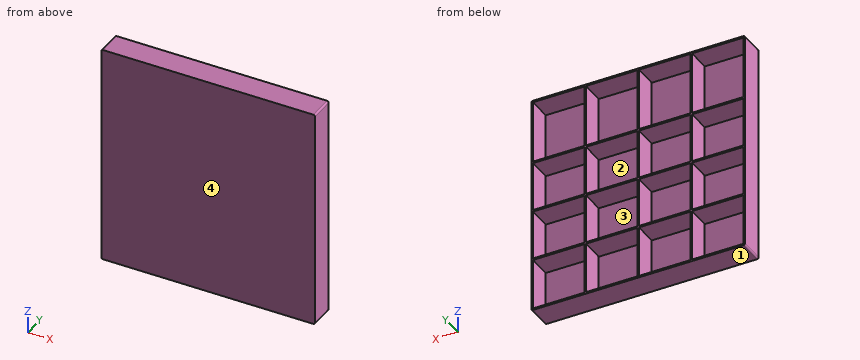
from build123d import *

# Parameters (mm, degrees)
SKETCH_1_W             = 258
SKETCH_1_H             = 268
EXTRUDE_1_DEPTH        = 2
SKETCH_2_W             = 258
SKETCH_2_H             = 268
SKETCH_2_W_2           = 254
SKETCH_2_H_2           = 264
EXTRUDE_2_DEPTH        = 28
SKETCH_3_W             = 2
SKETCH_3_H             = 264
EXTRUDE_3_DEPTH        = 28
PATTERN_LINEAR_1_COUNT = 3
PATTERN_LINEAR_1_PITCH = 64
SKETCH_4_W             = 254
SKETCH_4_H             = 2
EXTRUDE_5_DEPTH        = 28
PATTERN_LINEAR_2_COUNT = 3
PATTERN_LINEAR_2_PITCH = 62
FILLET_1_R             = 2


with BuildPart() as part:
    # 草图1 → 凸台-拉伸1 (new body)
    with BuildSketch(Plane(origin=(0, 0, 0), x_dir=(1, 0, 0), z_dir=(0, 1, 0))):
        Rectangle(SKETCH_1_W, SKETCH_1_H)
    extrude(amount=EXTRUDE_1_DEPTH)

    # 草图2 → 凸台-拉伸2 (add)
    with BuildSketch(Plane(origin=(0, 2, 0), x_dir=(1, 0, 0), z_dir=(0, 1, 0))):
        Rectangle(SKETCH_2_W, SKETCH_2_H)
        Rectangle(SKETCH_2_W_2, SKETCH_2_H_2, mode=Mode.SUBTRACT)
    extrude(amount=EXTRUDE_2_DEPTH)

    # 草图3 → 凸台-拉伸3 (add)
    with BuildSketch(Plane(origin=(0, 2, 0), x_dir=(1, 0, 0), z_dir=(0, 1, 0))):
        with Locations((-64, 0)):
            Rectangle(SKETCH_3_W, SKETCH_3_H)
    extrude_3 = extrude(amount=EXTRUDE_3_DEPTH)

    # 阵列(线性)1: 凸台-拉伸3 ×3
    with Locations(*[(i * PATTERN_LINEAR_1_PITCH, 0, 0) for i in range(1, PATTERN_LINEAR_1_COUNT)]):
        add(extrude_3)

    # 草图4 → 凸台-拉伸5 (add)
    with BuildSketch(Plane(origin=(0, 2, 0), x_dir=(1, 0, 0), z_dir=(0, 1, 0))):
        with Locations((0, 69)):
            Rectangle(SKETCH_4_W, SKETCH_4_H)
    extrude_5 = extrude(amount=EXTRUDE_5_DEPTH)

    # 阵列(线性)2: 凸台-拉伸5 ×3
    with Locations(*[(0, 0, i * PATTERN_LINEAR_2_PITCH) for i in range(1, PATTERN_LINEAR_2_COUNT)]):
        add(extrude_5)

    # 圆角1
    fillet_1_edges = [part.edges().sort_by_distance(p)[0] for p in [
        (-129, 15, -134),
        (129, 15, -134),
        (129, 15, 134),
        (-129, 15, 134),
    ]]
    fillet(fillet_1_edges, radius=FILLET_1_R)


solid = part.part
Work out the finished part from the listing and answer in its coordinate system (mm). Face numbers are marked on the shaded views. A direction names the side the tool comes from. Coordinates: 2 decimals unless noted, no trailing zeros. Write each loop counter-clockwise with the first axis right and the second up, starting at its lowest first coordinate (ties: lowest second). Pieces come first, ordered by that corner, then holes. Notation, with made-up numbers: M 26,0.25 L 84,0.25 A27 cw 84,37.25 Z; hole C -33.5,33.5 d10. An arc over 180 degrees is marked long. Use one line per item in the form item = value. Start each with the question number.
1. Each of these flat-tipped pins is pushed along its axis until it touches: P1, Ø8, axis at x = 79, z = -41.5, coming from the +Y side; P2, Ø12, axis at x = -38.5, z = -36.5, coming from the -Y side. Where does it stop, or does it pass through?
2. Straight lines are drawn through the part: probe 1 along Z at (x, y) = (-11, 15); probe 2 along X at (y, z) = (15.5, -102); probe 3 along Y at (x, z) = (113.5, -29). For each, find the intervals that lie inside material, in ascending order. Write a range as from..to.
3. A tool of negligible diameter and unlimited length cuts with its end or side. For the marked faces 3 and 4, from which of +Z, -Z, +X, -X, +Y, -Y can it reach the whole face along a straight path? Write none if from no direction.
4. The part is cut by section B-B (x = 17). Give the vertices of the cut face in (y, z), plus the area to 3 significant figures.
5. The part is cut by section A-A (z = -42). Give the vertices of the cut face in (x, y).
6. The mould has two halves that part along X. Classify the marked faces 1 and 2: released by +X, released by -X, zero draft, split by the parting line, or undercut.
7. The part is cut by section C-C (y = 22.5). Give the number of separate pieces and of enclosed holes in the cut face, plus the area to 3 significant figures.
Evaluation:
q1.P1 = 2
q1.P2 = 0
q2.probe_1 = -134..-132, -70..-68, -8..-6, 54..56, 132..134
q2.probe_2 = -129..-127, -65..-63, -1..1, 63..65, 127..129
q2.probe_3 = 0..2
q3.face_3 = +Y
q3.face_4 = +Z, -Z, +X, -X, -Y
q4.outline = M 0,-134 L 30,-134 L 30,-132 L 2,-132 L 2,-70 L 30,-70 L 30,-68 L 2,-68 L 2,-8 L 30,-8 L 30,-6 L 2,-6 L 2,54 L 30,54 L 30,56 L 2,56 L 2,132 L 30,132 L 30,134 L 0,134 Z
q4.area = 816 mm^2
q5.outline = M -129,0 L 129,0 L 129,30 L 127,30 L 127,2 L 65,2 L 65,30 L 63,30 L 63,2 L 1,2 L 1,30 L -1,30 L -1,2 L -63,2 L -63,30 L -65,30 L -65,2 L -127,2 L -127,30 L -129,30 Z
q6.face_1 = zero draft
q6.face_2 = undercut
q7.separate_pieces = 1
q7.enclosed_holes = 16
q7.area = 5,160 mm^2
